Part model, mm, in its own coordinate system. Coordinates: 2 decimals unless noted, no trailing zeros. Loops run counter-clockwise (first coordinate to the right, second up) from the corner with the lowest first, then second, coordinate; pieces in that order, holes last. Notation, with made-up numbers: (4.25, 10) -> (46.25, 10) arc R35 cw to (46.25, 46) -> close; hole circle Ø5 at (86, -1.5). An arc over 180 degrees is marked (long way). One line per item, written item: value. Start each with the question number.
from build123d import *

# Parameters (mm, degrees)
SKETCH1_R           = 25
BOSS_EXTRUDE1_DEPTH = 15
SKETCH2_R           = 25
BOSS_EXTRUDE2_DEPTH = 40
FILLET1_R           = 25


with BuildPart() as part:
    # Sketch1 → Boss-Extrude1 (new body)
    with BuildSketch(Plane(origin=(0, 0, 0), x_dir=(0, 0, -1), z_dir=(1, 0, 0))):
        Circle(SKETCH1_R)
        with BuildLine():
            Line((-2.5, 10), (2.5, 10))
            Line((2.5, 10), (2.5, 7.599342077))
            ThreePointArc((2.5, 7.599342077), (0, -8), (-2.5, 7.599342077))
            Line((-2.5, 7.599342077), (-2.5, 10))
        make_face(mode=Mode.SUBTRACT)
    extrude(amount=BOSS_EXTRUDE1_DEPTH)

    # Sketch2 → Boss-Extrude2 (add)
    with BuildSketch(Plane(origin=(15, 0, 0), x_dir=(0, 0, -1), z_dir=(1, 0, 0))):
        Circle(SKETCH2_R)
    extrude(amount=BOSS_EXTRUDE2_DEPTH)

    # Fillet1
    fillet1_edges = [part.edges().sort_by_distance(p)[0] for p in [
        (55, 0, 25),
    ]]
    fillet(fillet1_edges, radius=FILLET1_R)


solid = part.part
1) Slice it at A-A (x = 8). Give the cut face in (y, z).
2) Slice it at B-B (y = 0). Give the cut face in (x, z).
3) Probe line 1 (Y direction, x = 7, z = 0); line 2 (Z direction, x = 17, y = -20.5); line 3 (X direction, y = 18.5, z = -7). List the from-to ranges inside material, lowest first. Write a range as from..to.
4) Pull direction Z, two halves, no side cores. Call faces 1 (the cylindrical face through (14.79, 7.509, -23.846)), 2 (the flat face through (0, 6, 6)), 3 (the cylindrical face through (7, -8, 0)), 4 (the flat face through (7, 9, -2.5)): +Z half, -Z half, draft (parallel to the pull), parting line (faces both ways), or undercut.
5) Pin check, flat tips, straight feed: pin 1 Ø5 at (y, z) = (1, 14) entering from +X; pin 2 Ø1.2 at (x, y) = (8.5, 9) entering from +Z; pin 3 Ø1 at (y, z) = (12, -4.5) entering from +X. Stop position of each tip, or through.
6) Slice it at C-C (z = 0). Give the cut face in (x, y), then the cut area to 3 significant figures.
7) Slice it at D-D (x = 37). Give the cut face in (y, z), then the cut area to 3 significant figures.
Check sheet entries:
1. outline: circle Ø50 at (0, 0); hole (7.6, -2.5) -> (10, -2.5) -> (10, 2.5) -> (7.6, 2.5) arc R8 ccw (long way) to start
2. outline: (0, -25) -> (30, -25) arc R25 ccw to (30, 25) -> (0, 25) -> (0, 8) -> (15, 8) -> (15, -8) -> (0, -8) -> close
3. line 1: y = -25..-8, 10..25
3. line 2: z = -14.31..14.31
3. line 3: x = 0..45.29
4. face 1: parting line
4. face 2: draft
4. face 3: undercut
4. face 4: undercut
5. pin 1: stops at x = 52.18
5. pin 2: stops at z = 23.55
5. pin 3: stops at x = 51.76
6. outline: (0, -25) -> (30, -25) arc R25 ccw to (30, 25) -> (0, 25) -> (0, 10) -> (15, 10) -> (15, -8) -> (0, -8) -> close
6. area: 2,210 mm^2
7. outline: circle Ø48 at (0, 0)
7. area: 1,810 mm^2
